from build123d import *

# Parameters (mm, degrees)
BOSS_EXTRUDE1_DEPTH = 44.54
BOSS_EXTRUDE1_TAPER = -26.57
SKETCH2_OUTSIDE_W   = 156.308
SKETCH2_OUTSIDE_H   = 152.161
CUT_EXTRUDE1_DEPTH  = 44.54
CUT_EXTRUDE1_TAPER  = 26.57
SKETCH3_R           = 4.05
CUT_EXTRUDE2_DEPTH  = 35
SKETCH4_R           = 3.292788119
BOSS_EXTRUDE2_DEPTH = 130


with BuildPart() as part:
    # Sketch1 → Boss-Extrude1 (new body)
    with BuildSketch(Plane(origin=(0, 0, 0), x_dir=(1, 0, 0), z_dir=(0, 1, 0))):
        Polygon((0, 17.013016167), (-16.180339887, 5.257311121), (-10, -13.763819205), (10, -13.763819205), (16.180339887, 5.257311121), align=None)
    extrude(amount=BOSS_EXTRUDE1_DEPTH, taper=BOSS_EXTRUDE1_TAPER)

    # Sketch2 outside → Cut-Extrude1 (cut)
    with BuildSketch(Plane(origin=(0, 44.54, 0), x_dir=(1, 0, 0), z_dir=(0, 1, 0))):
        with Locations((0, 4.2535)):
            Rectangle(SKETCH2_OUTSIDE_W, SKETCH2_OUTSIDE_H)
        Polygon((0, -17.013016167), (16.180339887, -5.257311121), (10, 13.763819205), (-10, 13.763819205), (-16.180339887, -5.257311121), align=None, mode=Mode.SUBTRACT)
    extrude(amount=-CUT_EXTRUDE1_DEPTH, taper=CUT_EXTRUDE1_TAPER, mode=Mode.SUBTRACT)

    # Sketch3 → Cut-Extrude2 (cut)
    with BuildSketch(Plane(origin=(3.617528362, -6.155101222, 1.175406216), x_dir=(0.4408232334814932, 0.08851114782998275, -0.8932192639731522), z_dir=(0.49996506081853154, -0.8506735121122296, 0.16244849568822295))):
        with Locations(Location((1.971362597, 11.541364145, 0), (0, 0, 64.856110881))):
            Circle(SKETCH3_R)
    extrude(amount=-CUT_EXTRUDE2_DEPTH, mode=Mode.SUBTRACT)

    # Sketch4 → Boss-Extrude2 (add)
    with BuildSketch(Plane(origin=(-13.881248767, 23.618471702, -4.510291133), x_dir=(0.8660455749905556, 0.49109082304882484, -0.09378094452769076), z_dir=(0.49996506081853154, -0.8506735121122294, 0.16244849568822292))):
        with Locations(Location((10.937809574, 4.177759991, 0), (0, 0, 185.453817967))):
            Circle(SKETCH4_R)
    extrude(amount=BOSS_EXTRUDE2_DEPTH)


solid = part.part
The listing builds one solid part. Answer for the finished solid, in the listing's coordinates (mm). Give positions to 0.01 mm unless a question says otherwise; leave off trailing zeros. Use a Markdown table: item, result.
1. Section A-A on x = 7.5 is taken. Count the separate pieces of the cut face and the enclosed holes in it, plus the area to 3 significant figures.
Values follow:
| item | result |
|---|---|
| separate pieces | 2 |
| enclosed holes | 1 |
| area | 1,650 mm² |
2. Find the intervals of material crossed by probe 1 along Y at (x, z) = (-12, -6); probe 2 along Y at (x, z) = (-3, -2); probe 3 along X at (y, z) = (-4.5, 4), in increasing order. Write a range as from..to.
Values follow:
| item | result |
|---|---|
| probe 1 | y = 0..44.54 |
| probe 2 | y = 0..20.41, 21.91..44.54 |
| probe 3 | x = 12.03..19.2 |
3. Each of these flat-tipped pins is pushed along its axis until it touches: P1, Ø3, axis at x = 10, y = -2.5, coming from the +Z side; P2, Ø10, axis at y = 6, z = 3, coming from the +X side; P3, Ø2, axis at x = -10.5, y = 3, coming from the +Z side. Where does it stop, or does it pass through?
Values follow:
| item | result |
|---|---|
| P1 | stops at z = 6.62 |
| P2 | stops at x = 19.74 |
| P3 | stops at z = 15.76 |
4. For a pull along Z with two mould halves and no side action, classify faces 1 (the flat face through (-1, 0, -1)), 2 (the flat face through (60.63, -80.797, 19.64)), 3 (the cylindrical face through (1.9, 12.7, -0.98)) as released by +Z, released by -Z, zero draft, split by the parting line, or undercut.
Values follow:
| item | result |
|---|---|
| face 1 | zero draft |
| face 2 | released by +Z |
| face 3 | undercut |
